Autodesk Inventor part; units mm, degrees
ref_plane "Work Plane1" through (0, 0, -15) normal (0, 0, 1) x (1, 0, 0)
ref_plane "YZ Plane" through (0, 0, 0) normal (1, 0, 0) x (0, 1, 0)
ref_plane "XZ Plane" through (0, 0, 0) normal (0, 1, 0) x (-1, 0, 0)
sketch "Sketch1" plane through (0, 0, 0) normal (0, 0, 1) x (1, 0, 0)
  line L0 (0, 0) -> (25, 0)
  line L1 (25, 0) -> (25, 40)
  line L2 (25, 40) -> (0, 40)
  line L3 (0, 40) -> (0, 0)
  dimension "d1" = 25
  dimension "d2" = 40
  dimension "d3" = 25
extrude "Extrusion1" add sketch "Sketch1" against normal blind 30
sketch "Sketch2" plane through (25, 0, 0) normal (1, 0, 0) x (0, 0, -1)
  line L0 (0, 0) -> (30, 0)
  circle A0 centre (15, 6.56) radius 2.46
extrude "Extrusion2" cut sketch "Sketch2" against normal blind 30
sketch "Sketch3" plane through (0, 0, 0) normal (-1, 0, 0) x (0, 0, 1)
  line L0 (0, 0) -> (-30, 0)
  line L1 (-25.05, 0) -> (-4.95, 0)
  line L2 (-4.95, 0) -> (-4.95, 33.12)
  line L3 (-4.95, 33.12) -> (-25.05, 33.12)
  line L4 (-25.05, 33.12) -> (-25.05, 0)
  dimension "d11" = 20.1
extrude "Extrusion3" cut sketch "Sketch3" against normal blind 20
sketch "Sketch4" plane through (0, 0, 0) normal (0, -1, 0) x (1, 0, 0)
  line L0 (20, -4.95) -> (20, -25.05)
  line L1 (20, -15) -> (25, -15)
  line L2 (25, 0) -> (25, -30)
  line L3 (20, -8.025) -> (25, -8.025)
  line L4 (25, -8.025) -> (25, -21.975)
  line L5 (25, -21.975) -> (20, -21.975)
  line L6 (20, -21.975) -> (20, -8.025)
  line L7 (20, -8.025) -> (25, -21.975) construction
  line L8 (25, -8.025) -> (20, -21.975) construction
  line L9 (25, -12.54) -> (25, -17.46)
  point P0 (0, 0)
  point P1 (22.5, -15)
  dimension "d14" = 13.95
extrude "Extrusion4" add sketch "Sketch4" along normal blind 15
sketch "Sketch5" plane through (20, 0, 0) normal (-1, 0, 0) x (0, 0, 1)
  circle A0 centre (-15, 6.56) radius 2.46
  circle A1 centre (-15, 6.56) radius 4.7025
  circle A2 centre (-15, 6.56) radius 2.46
  circle A3 centre (-15, 6.56) radius 2.46
  point P0 (0, 0)
  dimension "d17" = 9.405
extrude "Extrusion5" cut sketch "Sketch5" against normal blind 2.1
sketch "Sketch6" plane through (25, 0, 0) normal (1, 0, 0) x (0, 0, -1)
  circle A0 centre (15, 6.56) radius 4.7025
  line L0 (15, 6.56) -> (15, 23.56)
  circle A1 centre (15, 23.56) radius 2.46
  point P0 (0, 0)
  dimension "d20" = 17
  dimension "d21" = 4.92
extrude "Extrusion6" cut sketch "Sketch6" against normal blind 10 contours A1
sketch "Sketch7" plane through (20, 0, 0) normal (-1, 0, 0) x (0, 0, 1)
  circle A0 centre (-15, 23.56) radius 2.46
  circle A1 centre (-15, 23.56) radius 4.7025
  point P0 (0, 0)
  dimension "d24" = 9.405
extrude "Extrusion7" cut sketch "Sketch7" against normal blind 2.1
sketch "Sketch9" plane through (25, 0, 0) normal (1, 0, 0) x (0, 0, -1)
  circle A0 centre (15, 6.56) radius 2.46
  circle A1 centre (15, 6.56) radius 2.46
  circle A2 centre (15, 23.56) radius 2.46
  circle A3 centre (15, 23.56) radius 2.46
  line L0 (30, 40) -> (30, 0)
  line L1 (30, 0) -> (30, 40)
  line L2 (30, 40) -> (0, 40)
  line L3 (0, 40) -> (0, 0)
  line L4 (0, 0) -> (8.025, 0)
  line L5 (21.975, 0) -> (21.975, -15)
  line L6 (21.975, -15) -> (8.025, -15)
  line L7 (8.025, -15) -> (8.025, 0)
  line L8 (0, 0) -> (8.025, 0)
  line L9 (21.975, 0) -> (30, 0)
extrude "Extrusion8" add sketch "Sketch9" along normal blind 5
sketch "Sketch10" plane through (0, 40, 0) normal (0, 1, 0) x (1, 0, 0)
  line L0 (0, 30) -> (30, 30)
  line L1 (30, 0) -> (0, 0)
  line L2 (0, 30) -> (30, 30)
  line L3 (30, 30) -> (30, 0)
  line L4 (30, 0) -> (0, 0)
  line L5 (0, 0) -> (0, 30)
extrude "Extrusion9" add sketch "Sketch10" along normal blind 30
sketch "Sketch12" plane through (30, 0, 0) normal (1, 0, 0) x (0, 0, -1)
  circle A0 centre (15, 6.56) radius 2.46
  line L0 (15, 6.56) -> (15, 15.06)
  circle A1 centre (15, 15.06) radius 2.525
  point P0 (0, 0)
  dimension "d31" = 8.5
  dimension "d33" = 5.05
extrude "Extrusion10" cut sketch "Sketch12" against normal blind 30 contours A1
sketch "Sketch14" plane through (0, 0, 0) normal (0, 0, 1) x (1, 0, 0)
  line L0 (30, 70) -> (0, 70)
  line L1 (0, 70) -> (0, 85)
  line L2 (-15, 100) -> (-23, 100)
  line L3 (30, 0) -> (30, 70)
  line L4 (30, 122.5) -> (30, 70)
  arc A0 (0, 85) -> (-15, 100) centre (-15, 85) ccw
  line L5 (30, 105) -> (30, 100)
  line L6 (-23, 153) -> (15, 153)
  line L7 (-18, 150.5) -> (-23, 153)
  line L8 (-18, 102.5) -> (-23, 100)
  line L9 (-18, 102.5) -> (-13, 126.5)
  line L10 (-13, 126.5) -> (-18, 150.5)
  line L11 (30, 126.5) -> (15, 153)
  line L12 (30, 122.5) -> (30, 126.5)
  point P0 (0, 0)
  point P1 (0, 100)
  dimension "d47" = 30
  dimension "d54" = 15
extrude "Extrusion12" add sketch "Sketch14" against normal blind 30
sketch "Sketch15" plane through (0, 0, -25.05) normal (-1, 0, 0) x (0, 0, 1)
  line L0 (0, 33.12) -> (20.1, 33.12)
  line L1 (20.1, 33.12) -> (20.1, 0)
  line L2 (0, 33.12) -> (20.1, 33.12)
  line L3 (20.1, 33.12) -> (20.1, 31.1)
  line L4 (20.1, 31.1) -> (0, 31.1)
  line L5 (0, 31.1) -> (0, 33.12)
  point P0 (25.05, 0)
  dimension "d57" = 2.02
extrude "Extrusion13" add sketch "Sketch15" against normal blind 20
sketch "Sketch25" plane through (0, 0, 0) normal (0, 0, 1) x (1, 0, 0)
  line L0 (-15, 100) -> (-23, 100)
  line L1 (-15, 100) -> (-23, 100)
  line L2 (-23, 100) -> (-18, 102.5)
  line L3 (-23, 100) -> (-18, 102.5)
  line L4 (-18, 102.5) -> (-13, 126.5)
  line L5 (-18, 102.5) -> (-13, 126.5)
  line L6 (-13, 126.5) -> (-18, 150.5)
  line L7 (-13, 126.5) -> (-18, 150.5)
  line L8 (-18, 150.5) -> (-23, 153)
  line L9 (-18, 150.5) -> (-23, 153)
  line L10 (-23, 153) -> (15, 153)
  line L11 (-23, 153) -> (15, 153)
  line L12 (15, 153) -> (30, 126.5)
  line L13 (15, 153) -> (30, 126.5)
  line L14 (30, 126.5) -> (30, 76.5)
  line L15 (30, 0) -> (30, 126.5)
  line L16 (30, 76.5) -> (0, 76.5)
  arc A0 (0, 85) -> (-15, 100) centre (-15, 85) ccw
  line L17 (0, 76.5) -> (0, 85)
  line L18 (0, 85) -> (0, 0)
  arc A1 (0, 85) -> (-15, 100) centre (-15, 85) ccw
  dimension "d90" = 50
extrude "Extrusion14" add sketch "Sketch25" along normal blind 15
ref_plane "Work Plane1" through (0, 0, -15) normal (0, 0, 1) x (1, 0, 0)
mirror "Mirror1" about plane through (0, 0, -15) normal (0, 0, 1) of "Extrusion14"
properties part number "rec_a_48mm_x_60mm"
Verification items for the finished model (mm, model axes). A direction names the side the tool comes from. Coordinates: 2 decimals unless noted, no trailing zeros. Loops run counter-clockwise (first coordinate to the right, second up) from the corner with the lowest first, then second, coordinate; pieces in that order, holes last. Notation, with made-up numbers: (72.5, 37.5) -> (93.5, 37.5) arc R19 ccw to (93.5, 57.5) -> close; hole circle Ø6 at (44.5, 70.5). An arc over 180 degrees is marked (long way). Put each result on its own line as item: value.
1. Mould release check, pull along Z, two halves, no side actions. Record for faces 4 (the face through (-20.465, 101.268, -14.58)), 5 (the face through (25, -7, -21.975)), 6 (the face through (25.995, 24.502, -17.272)), 7 (the face through (15, 39, 0)): pulls with the +Z half, pulls with the -Z half, needs draft (parallel to the pull), parting line crosses it, or undercut.
Result set:
face 4: needs draft
face 5: pulls with the -Z half
face 6: undercut
face 7: pulls with the +Z half
2. Section check B-B, the plane x = 25.5. Record the boundary of the cut face in (y, z) (3 decimals).
Result set:
outline: (-15, -21.975) -> (0, -21.975) -> (0, -30) -> (76.5, -30) -> (76.5, -45) -> (134.45, -45) -> (134.45, 15) -> (76.5, 15) -> (76.5, 0) -> (0, 0) -> (0, -8.025) -> (-15, -8.025) -> close; hole circle Ø4.92 at (6.56, -15); hole circle Ø5.05 at (15.06, -15); hole circle Ø4.92 at (23.56, -15)
3. Gauge pin test, flat ends, axial feed: P1, Ø4.5, axis at y = 24, z = -16.5, coming from the -X side; P2, Ø4, axis at x = 23.5, y = 54, coming from the +Z side; P3, Ø10, axis at x = 1.5, y = 69, coming from the -Z side; P4, Ø5.5, axis at y = 23.56, z = -15, coming from the +X side. Record the tip position at first contact, or that the pin passes through.
Result set:
P1: stops at x = 22.1
P2: stops at z = 0
P3: stops at z = -30
P4: stops at x = 30
4. Thickness scan on line 1 (Y direction, x = 27.75, z = -15) (3 decimals); line 2 (Y direction, x = 24, z = -15) (3 decimals); line 3 (X direction, y = 100.5, z = -12). Record the ranges inside material, lowest first.
Result set:
line 1: y = -15 to 4.1, 9.02 to 12.535, 17.585 to 21.1, 26.02 to 130.475
line 2: y = -15 to 4.1, 9.02 to 12.535, 17.585 to 21.1, 26.02 to 137.1
line 3: x = -22 to 30
5. Section check D-D, the plane z = -40.5. Record the boundary of the cut face in (x, y), then the cut area to 3 significant figures.
Result set:
outline: (-23, 100) -> (-15, 100) arc R15 cw to (0, 85) -> (0, 76.5) -> (30, 76.5) -> (30, 126.5) -> (15, 153) -> (-23, 153) -> (-18, 150.5) -> (-13, 126.5) -> (-18, 102.5) -> close
area: 2,990 mm^2
6. Section check C-C, the plane y = 15.06. Record the boundary of the cut face in (x, z) (3 decimals), then the cut area to 4 significant figures.
Result set:
outline: (0, -30) -> (30, -30) -> (30, -17.525) -> (20, -17.525) -> (20, -25.05) -> (0, -25.05) -> close; (0, -4.95) -> (20, -4.95) -> (20, -12.475) -> (30, -12.475) -> (30, 0) -> (0, 0) -> close
area: 447.5 mm^2
7. Tool access check on faces 1 (the face through (0, 53, -15)), 2 (the face through (15, 76.5, 7)), 3 (the face through (21.035, 7.973, -10.515)). Record the directions out of +Z, -Z, +X, -X, +Y, -Y that give a thin tool (end or side, any length) a straight path to the whole face; none if there is none.
Result set:
face 1: +Z, -Z, -X, -Y
face 2: +Z, +X, -X, -Y
face 3: -X
8. Section check A-A, the plane z = -15. Give the number of separate pieces and of enclosed holes in the cut face, then the cut area to 3 significant figures.
Result set:
separate pieces: 4
enclosed holes: 0
area: 4,650 mm^2
